```python
from build123d import *

# Parameters (mm, degrees)
SKETCH_1_W           = 87
SKETCH_1_H           = 50
SKETCH_1_R           = 1.6
EXTRUDE_1_DEPTH      = 1.5
EXTRUDE_2_DEPTH      = 4
EXTRUDE_2_DEPTH_BACK = 12
SKETCH_2_W           = 74
SKETCH_2_H           = 50
SKETCH_3_W           = 58
SKETCH_3_H           = 40
EXTRUDE_3_DEPTH      = 22


with BuildPart() as part:
    # 草图1 → 凸台-拉伸1 (new body)
    with BuildSketch(Plane(origin=(0, 0, 0), x_dir=(1, 0, 0), z_dir=(0, 1, 0))):
        Rectangle(SKETCH_1_W, SKETCH_1_H)
        with Locations(Location((-39.5, 21, 0), (0, 0, 270))):
            Circle(SKETCH_1_R, mode=Mode.SUBTRACT)
        with Locations(Location((-39.5, -21, 0), (0, 0, 90))):
            Circle(SKETCH_1_R, mode=Mode.SUBTRACT)
        with Locations(Location((39.5, -21, 0), (0, 0, 270))):
            Circle(SKETCH_1_R, mode=Mode.SUBTRACT)
        with Locations(Location((39.5, 21, 0), (0, 0, 90))):
            Circle(SKETCH_1_R, mode=Mode.SUBTRACT)
    extrude(amount=EXTRUDE_1_DEPTH)

    # 草图2 → 凸台-拉伸2 (add, two sides: drawn at the far end of the back side and taken through both)
    with BuildSketch(Plane.XZ.offset(-EXTRUDE_2_DEPTH_BACK)):
        Rectangle(SKETCH_2_W, SKETCH_2_H)
    extrude(amount=EXTRUDE_2_DEPTH + EXTRUDE_2_DEPTH_BACK)

    # 草图3 → 凸台-拉伸3 (add)
    with BuildSketch(Plane(origin=(0, 12, 0), x_dir=(1, 0, 0), z_dir=(0, 1, 0))):
        with Locations((0, 4)):
            Rectangle(SKETCH_3_W, SKETCH_3_H)
    extrude(amount=EXTRUDE_3_DEPTH)


solid = part.part
```
Geometry check sheet. Reference: the model listing, model coordinates, mm. A direction names the side the tool comes from. Coordinates: 2 decimals unless noted, no trailing zeros. Order: outer loops, then holes, each group sorted by start corner. A loop starts at its lowest first (then second) coordinate and runs counter-clockwise, first axis right, second up. Notation, with made-up numbers: M 9,64.5 L 55,64.5 A26 ccw 55,98.5 Z; hole C 55.25,-13.75 d9. An arc over 180 degrees is marked long. Answer as a JSON object with one key per item and string values.
Q1. Depth check by flat-ended pin: pin 1 Ø6 at (x, y) = (-15, 18) entering from +Z; pin 2 Ø2 at (x, z) = (-40.5, 12) entering from +Y; pin 3 Ø1.2 at (y, z) = (-2.5, 6.5) entering from +X; pin 4 Ø1.9 at (x, z) = (-39.5, 21) entering from +Y. Enter the tip coordinate at first touch or a pass-through.
Results are:
{"pin 1": "stops at z = 16", "pin 2": "stops at y = 1.5", "pin 3": "stops at x = 37", "pin 4": "passes through"}
Q2. Scan lines: line 1 (Y direction, x = -31, z = -21.5); line 2 (X direction, y = 5.5, z = -6); line 3 (Y direction, x = 40, z = -2). Record each from-to range of solid material in increasing order.
Results are:
{"line 1": "y = -4 to 12", "line 2": "x = -37 to 37", "line 3": "y = 0 to 1.5"}
Q3. Release check for a two-part mould opening along X. For faces 1 (the cylindrical face through (41.06, 0.74, -20.65)), 2 (the flat face through (-1, -4, 0)), 3 (the flat face through (-37, -2, 0)) record: released by +X, released by -X, zero draft, split by the parting line, or undercut.
Results are:
{"face 1": "undercut", "face 2": "zero draft", "face 3": "released by -X"}
Q4. Cross-section at C-C on x = -9. Record the cut outline in (y, z), and give its area (3 significant figures).
Results are:
{"outline": "M -4,-25 L 12,-25 L 12,-24 L 34,-24 L 34,16 L 12,16 L 12,25 L -4,25 Z", "area": "1,680 mm²"}
Q5. Cross-section at A-A on z = -21. Record the cut outline in (x, y).
Results are:
{"outline": "M -43.5,0 L -41.1,0 L -41.1,1.5 L -43.5,1.5 Z; M -37.9,0 L -37,0 L -37,-4 L 37,-4 L 37,0 L 37.9,0 L 37.9,1.5 L 37,1.5 L 37,12 L 29,12 L 29,34 L -29,34 L -29,12 L -37,12 L -37,1.5 L -37.9,1.5 Z; M 41.1,0 L 43.5,0 L 43.5,1.5 L 41.1,1.5 Z"}
Q6. Cross-section at D-D on z = 21. Record the cut outline in (x, y).
Results are:
{"outline": "M -43.5,0 L -41.1,0 L -41.1,1.5 L -43.5,1.5 Z; M -37.9,0 L -37,0 L -37,-4 L 37,-4 L 37,0 L 37.9,0 L 37.9,1.5 L 37,1.5 L 37,12 L -37,12 L -37,1.5 L -37.9,1.5 Z; M 41.1,0 L 43.5,0 L 43.5,1.5 L 41.1,1.5 Z"}
Q7. Tool access check on faces 4 (the flat face through (37, -2, 0)), 5 (the flat face through (37, 7, 0)), 6 (the flat face through (-40, 0, 0)), 7 (the flat face through (0, 23, -24)). Record the directions out of +Z, -Z, +X, -X, +Y, -Y that give a thin tool (end or side, any length) a straight path to the whole face; none if there is none.
Results are:
{"face 4": "+Z, -Z, +X, -Y", "face 5": "+Z, -Z, +X, +Y", "face 6": "+Z, -Z, -X, -Y", "face 7": "-Z, +X, -X, +Y"}
Q8. Cross-section at B-B on x = 39.5. Record the cut outline in (y, z).
Results are:
{"outline": "M 0,-25 L 1.5,-25 L 1.5,-22.6 L 0,-22.6 Z; M 0,-19.4 L 1.5,-19.4 L 1.5,19.4 L 0,19.4 Z; M 0,22.6 L 1.5,22.6 L 1.5,25 L 0,25 Z"}
